Design review of the part built by this model. Coordinates are the model's own, in mm. Face numbers are marked on the shaded views. Round coordinates to 2 decimals unless told otherwise and drop trailing zeros. Order: outer loops, then holes, each group sorted by start corner. A loop starts at its lowest first (then second) coordinate and runs counter-clockwise, first axis right, second up. Notation, with made-up numbers: M 7,56.5 L 46,56.5 A34 cw 46,87.5 Z; hole C 72,89 d4. An arc over 180 degrees is marked long. Use a Markdown table: item, result. Add a question column.
(1) To check wall thickness, follow probe 1 along Y at (x, z) = (5, -1.85); probe 2 along Y at (x, z) = (2.5, -4.75); probe 3 along X at (y, z) = (31.5, -0.25) (3 decimals). State the ranges of each line that lie inside material, in increasing order. Write a range as from..to.
(2) Take a section at C-C (y = -26.5). Write out the cut boundary in (x, z) (3 decimals).
(3) The part is to be moulded in two halves that separate along Y. For the marked faces 1 and 2, say which applies: released by +Y, released by -Y, zero draft, split by the parting line, or undercut.
(4) For pin 1 (1.5 mm diameter, centred on x = 6, z = -2, fed in from -Y); pin 2 (1.6 mm diameter, centred on x = 9.25, y = -87, fed in from -Z); pin 3 (1.8 mm diameter, centred on y = 21.5, z = -3, fed in from +X) (3 decimals); pin 4 (1.8 mm diameter, centred on y = 31, z = -3.5, fed in from +X) (3 decimals), all flat-tipped, find the tip position at first contact; note any pin that passes through.
(5) Take a section at A-A (y = 62). Write out the cut boundary in (x, z) (3 decimals), then the cut area to 4 significant figures.
(6) Take a section at B-B (z = -2). Count the separate pieces of the cut face and the enclosed holes in it, then the cut area to 3 significant figures.
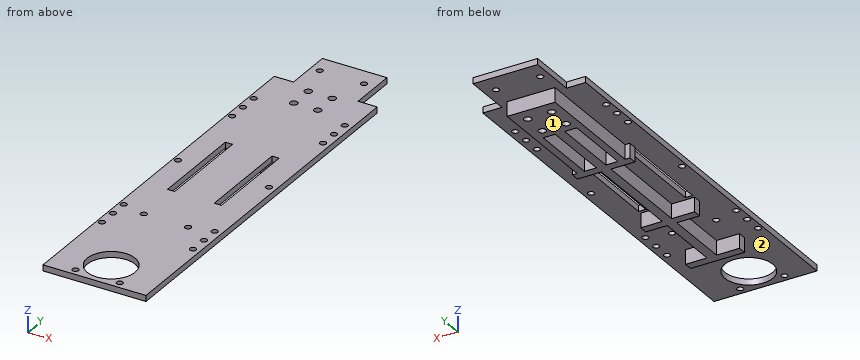
```python
from build123d import *

# Parameters (mm, degrees)
SKETCH_1_R      = 1.3
SKETCH_1_R_2    = 10
SKETCH_1_W      = 3
SKETCH_1_H      = 40
SKETCH_1_R_3    = 1.55
EXTRUDE_1_DEPTH = 2.5
SKETCH_2_R      = 1.55
SKETCH_2_W      = 3
SKETCH_2_H      = 28.5
SKETCH_2_W_2    = 4
SKETCH_2_H_2    = 27.5
SKETCH_2_W_3    = 9.575
SKETCH_2_H_3    = 3.5
SKETCH_2_W_4    = 8.925
EXTRUDE_2_DEPTH = 6


with BuildPart() as part:
    # 草图1 → 凸台-拉伸1 (new body)
    with BuildSketch(Plane.XY):
        Polygon((22, -90), (22, 70), (14, 70), (14, 90), (-13, 90), (-13, 70), (-21, 70), (-21, -90), (-16, -90), (-2.5, -90), (2.5, -90), (16, -90), align=None)
        with Locations((-19, -52.5)):
            Circle(SKETCH_1_R, mode=Mode.SUBTRACT)
        with Locations((-9.25, -87)):
            Circle(SKETCH_1_R, mode=Mode.SUBTRACT)
        with Locations((0, -77.615961472)):
            Circle(SKETCH_1_R_2, mode=Mode.SUBTRACT)
        with Locations((-19, -45)):
            Circle(SKETCH_1_R, mode=Mode.SUBTRACT)
        with Locations((-19, -37.5)):
            Circle(SKETCH_1_R, mode=Mode.SUBTRACT)
        with Locations((-9.25, -39.714835276)):
            Circle(SKETCH_1_R, mode=Mode.SUBTRACT)
        with Locations((9.25, -87)):
            Circle(SKETCH_1_R, mode=Mode.SUBTRACT)
        with Locations((19, -52.5)):
            Circle(SKETCH_1_R, mode=Mode.SUBTRACT)
        with Locations((9.25, -39.714835276)):
            Circle(SKETCH_1_R, mode=Mode.SUBTRACT)
        with Locations((19, -45)):
            Circle(SKETCH_1_R, mode=Mode.SUBTRACT)
        with Locations((19, -37.5)):
            Circle(SKETCH_1_R, mode=Mode.SUBTRACT)
        with Locations((-19, 0)):
            Circle(SKETCH_1_R, mode=Mode.SUBTRACT)
        with Locations((-19, 37.5)):
            Circle(SKETCH_1_R, mode=Mode.SUBTRACT)
        with Locations((-9.75, 0)):
            Rectangle(SKETCH_1_W, SKETCH_1_H, mode=Mode.SUBTRACT)
        with Locations((-19, 45)):
            Circle(SKETCH_1_R, mode=Mode.SUBTRACT)
        with Locations((-19, 52.5)):
            Circle(SKETCH_1_R, mode=Mode.SUBTRACT)
        with Locations((-5, 57)):
            Circle(SKETCH_1_R_3, mode=Mode.SUBTRACT)
        with Locations((-5, 67)):
            Circle(SKETCH_1_R_3, mode=Mode.SUBTRACT)
        with Locations((-9.25, 82)):
            Circle(SKETCH_1_R, mode=Mode.SUBTRACT)
        with Locations((9.75, 0)):
            Rectangle(SKETCH_1_W, SKETCH_1_H, mode=Mode.SUBTRACT)
        with Locations((19, 0)):
            Circle(SKETCH_1_R, mode=Mode.SUBTRACT)
        with Locations((19, 37.5)):
            Circle(SKETCH_1_R, mode=Mode.SUBTRACT)
        with Locations((5, 57)):
            Circle(SKETCH_1_R_3, mode=Mode.SUBTRACT)
        with Locations((5, 67)):
            Circle(SKETCH_1_R_3, mode=Mode.SUBTRACT)
        with Locations((9.25, 82)):
            Circle(SKETCH_1_R, mode=Mode.SUBTRACT)
        with Locations((19, 45)):
            Circle(SKETCH_1_R, mode=Mode.SUBTRACT)
        with Locations((19, 52.5)):
            Circle(SKETCH_1_R, mode=Mode.SUBTRACT)
    extrude(amount=EXTRUDE_1_DEPTH)

    # 草图2 → 凸台-拉伸2 (add)
    with BuildSketch(Plane(origin=(0, 0, 0), x_dir=(-1, 0, 0), z_dir=(0, 0, -1))):
        Polygon((9.675, 72.5), (9.675, 52.5), (1.675, 52.5), (-0.325, 52.5), (-2.325, 52.5), (-10.325, 52.5), (-10.325, 72.5), align=None)
        with Locations((-5, 57)):
            Circle(SKETCH_2_R, mode=Mode.SUBTRACT)
        with Locations((5, 67)):
            Circle(SKETCH_2_R, mode=Mode.SUBTRACT)
        with Locations((-5, 67)):
            Circle(SKETCH_2_R, mode=Mode.SUBTRACT)
        with Locations((5, 57)):
            Circle(SKETCH_2_R, mode=Mode.SUBTRACT)
        with Locations((8.175, 38.25)):
            Rectangle(SKETCH_2_W, SKETCH_2_H)
        Polygon((-2.325, 20.5), (1.675, 20.5), (1.675, 24), (1.675, 32.5), (1.675, 52.5), (-0.325, 52.5), (-2.325, 52.5), (-2.325, 32.5), (-2.325, 24), align=None)
        with Locations((-8.825, 38.25)):
            Rectangle(SKETCH_2_W, SKETCH_2_H)
        Polygon((-12.325, 20.5), (-2.325, 20.5), (-2.325, 24), (-7.325, 24), (-10.325, 24), (-12.325, 24), align=None)
        Polygon((1.675, 24), (1.675, 20.5), (11.675, 20.5), (11.675, 24), (9.675, 24), (6.675, 24), align=None)
        Polygon((-2.325, 20), (-2.325, -21.5), (1.675, -21.5), (1.675, 20.5), (-2.325, 20.5), align=None)
        with Locations((-0.325, -38.75)):
            Rectangle(SKETCH_2_W_2, SKETCH_2_H_2)
        with Locations((6.4625, -23.25)):
            Rectangle(SKETCH_2_W_3, SKETCH_2_H_3)
        with Locations((-0.325, -23.25)):
            Rectangle(SKETCH_2_W_2, SKETCH_2_H_3)
        with Locations((-6.7875, -23.25)):
            Rectangle(SKETCH_2_W_4, SKETCH_2_H_3)
        Polygon((-11.25, -52.5), (-2.325, -52.5), (1.675, -52.5), (11.25, -52.5), (11.25, -56), (-11.25, -56), align=None)
    extrude(amount=EXTRUDE_2_DEPTH)


solid = part.part
```
Verdict:
| question | item | result |
|---|---|---|
| 1 | probe 1 | y = -56..-52.5, -25..-21.5, 20.5..24, 52.5..55.45, 58.55..65.45, 68.55..72.5 |
| 1 | probe 2 | y = -56..-52.5, -25..-21.5, 20.5..24, 52.5..72.5 |
| 1 | probe 3 | x = -9.675..-6.675, -1.675..2.325, 7.325..10.325 |
| 2 | outline | M -21,0 L -1.675,0 L -1.675,-6 L 2.325,-6 L 2.325,0 L 22,0 L 22,2.5 L -21,2.5 Z |
| 3 | face 1 | zero draft |
| 3 | face 2 | undercut |
| 4 | pin 1 | stops at y = -56 |
| 4 | pin 2 | passes through |
| 4 | pin 3 | stops at x = 12.325 |
| 4 | pin 4 | stops at x = 10.325 |
| 5 | outline | M -21,0 L -9.675,0 L -9.675,-6 L 10.325,-6 L 10.325,0 L 22,0 L 22,2.5 L -21,2.5 Z |
| 5 | area | 227.5 mm^2 |
| 6 | separate pieces | 1 |
| 6 | enclosed holes | 6 |
| 6 | area | 1,170 mm^2 |
